from build123d import *

# Parameters (mm, degrees)
SKETCH1_W           = 110
SKETCH1_H           = 10
SKETCH1_W_2         = 10
SKETCH1_H_2         = 250
BOSS_EXTRUDE1_DEPTH = 50
FILLET1_R           = 10
SKETCH2_R           = 4
CUT_EXTRUDE1_DEPTH  = 149
SKETCH3_R           = 10
CUT_EXTRUDE2_DEPTH  = 10


with BuildPart() as part:
    # Sketch1 → Boss-Extrude1 (new body)
    with BuildSketch(Plane.XY):
        with Locations((65, -5)):
            Rectangle(SKETCH1_W, SKETCH1_H)
        with Locations((5, -125)):
            Rectangle(SKETCH1_W_2, SKETCH1_H_2)
        Polygon((130, 0), (120, 0), (120, -10), (120, -250), (130, -250), align=None)
    extrude(amount=BOSS_EXTRUDE1_DEPTH)

    # Fillet1
    fillet1_edges = [part.edges().sort_by_distance(p)[0] for p in [
        (0, 0, 25),
        (130, 0, 25),
    ]]
    fillet(fillet1_edges, radius=FILLET1_R)

    # Sketch2 → Cut-Extrude1 (cut)
    with BuildSketch(Plane(origin=(130, 0, 0), x_dir=(0, 0, -1), z_dir=(1, 0, 0))):
        with Locations(Location((-25, -225, 0), (0, 0, 90))):
            Circle(SKETCH2_R)
    extrude(amount=-CUT_EXTRUDE1_DEPTH, mode=Mode.SUBTRACT)

    # Sketch3 → Cut-Extrude2 (cut)
    with BuildSketch(Plane(origin=(0, 0, 0), x_dir=(1, 0, 0), z_dir=(0, 1, 0))):
        with Locations(Location((65, -25, 0), (0, 0, 270))):
            Circle(SKETCH3_R)
    extrude(amount=-CUT_EXTRUDE2_DEPTH, mode=Mode.SUBTRACT)


solid = part.part
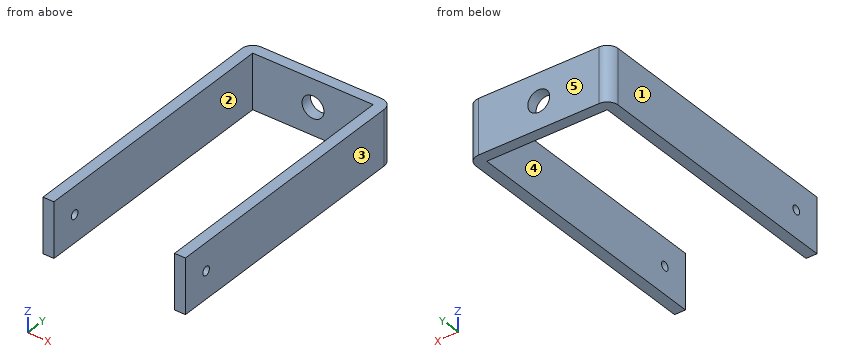
Verification items for the finished model (mm, model axes). Face numbers are marked on the shaded views. A direction names the side the tool comes from. Give positions to 0.01 mm unless a question says otherwise; leave off trailing zeros. Write each loop counter-clockwise with the first axis right and the second up, starting at its lowest first coordinate (ties: lowest second). Pieces come first, ordered by that corner, then holes. Notation, with made-up numbers: (12, 43) -> (66, 43) arc R30 ccw to (66, 75) -> close; hole circle Ø8 at (36.5, 76). An arc over 180 degrees is marked (long way). Use CSV: the item, a comma, the result in double quotes.
(1) Material ranges on L1, parallel to Z at x = 3, y = -225; L2, parallel to X at y = -61.5, z = 18.5; L3, parallel to Y at x = 98, z = 31.5, recorded low to high.
Derived:
L1,"z = 0 to 21, 29 to 50"
L2,"x = 0 to 10, 120 to 130"
L3,"y = -10 to 0"
(2) Go/stop test with flat-tipped pins: pin 1 (4 mm diameter, centred on x = 40.5, z = 44, fed in from -Y); pin 2 (13 mm diameter, centred on y = -225, z = 25, fed in from -X). Record where each tip stops, or that it passes through.
Derived:
pin 1,"stops at y = -10"
pin 2,"stops at x = 0"
(3) Sectioned sample at C-C (y = -225). Record the cut outline in (x, z), plus the area to 3 significant figures.
Derived:
outline,"(0, 0) -> (10, 0) -> (10, 21) -> (0, 21) -> close; (0, 29) -> (10, 29) -> (10, 50) -> (0, 50) -> close; (120, 0) -> (130, 0) -> (130, 21) -> (120, 21) -> close; (120, 29) -> (130, 29) -> (130, 50) -> (120, 50) -> close"
area,"840 mm^2"
(4) Sectioned sample at D-D (x = 65). Record the cut outline in (y, z).
Derived:
outline,"(-10, 0) -> (0, 0) -> (0, 15) -> (-10, 15) -> close; (-10, 35) -> (0, 35) -> (0, 50) -> (-10, 50) -> close"
(5) Sectioned sample at A-A (z = 25). Record the cut outline in (x, y).
Derived:
outline,"(0, -250) -> (10, -250) -> (10, -229) -> (0, -229) -> close; (0, -221) -> (10, -221) -> (10, -10) -> (55, -10) -> (55, 0) -> (10, 0) arc R10 ccw to (0, -10) -> close; (75, -10) -> (120, -10) -> (120, -221) -> (130, -221) -> (130, -10) arc R10 ccw to (120, 0) -> (75, 0) -> close; (120, -250) -> (130, -250) -> (130, -229) -> (120, -229) -> close"
(6) Sectioned sample at B-B (y = -118.5). Record the cut outline in (x, z).
Derived:
outline,"(0, 0) -> (10, 0) -> (10, 50) -> (0, 50) -> close; (120, 0) -> (130, 0) -> (130, 50) -> (120, 50) -> close"
(7) Release check for a two-part mould opening along X. For the marked faces 1, 2 and 3 record: +X half, -X half, draft (parallel to the pull), parting line (faces both ways), or undercut.
Derived:
face 1,"-X half"
face 2,"undercut"
face 3,"+X half"
(8) Set-up check for the marked faces 4 and 5: record each of +Z, -Z, +X, -X, +Y, -Y from which the full face is reachable in a straight line by a thin tool's end or side.
Derived:
face 4,"+Z, -Z, -Y"
face 5,"+Z, -Z, +X, -X, +Y"
